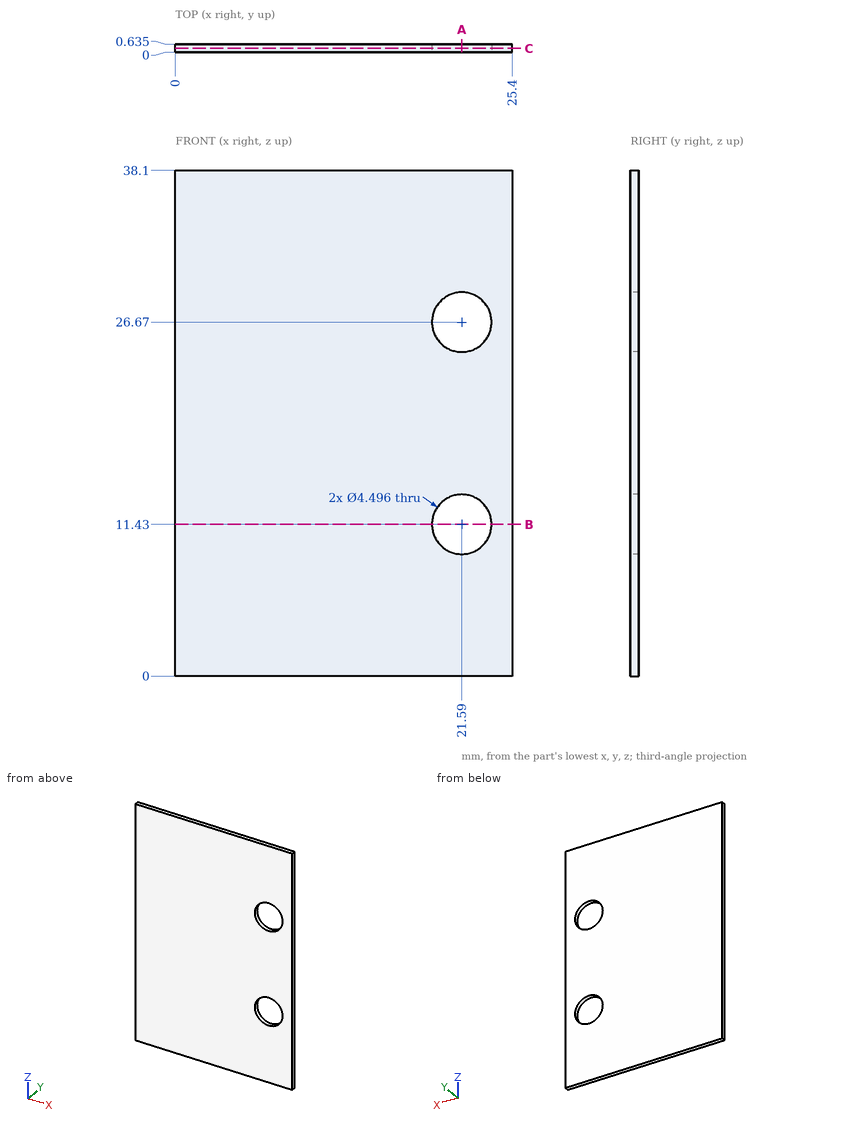
Check sheet for the drawn part. Datum: minimum x, y, z corner. Units: mm. Coordinates: 2 decimals unless noted, no trailing zeros. Order: outer loops, then holes, each group sorted by start corner. A loop starts at its lowest first (then second) coordinate and runs counter-clockwise, first axis right, second up. Notation, with made-up numbers: M 58.5,4 L 100.5,4 A5 ccw 100.5,10 Z; hole C 74.5,15 d9. An arc over 180 degrees is marked long. One line per question, with ' | ' between items. Start each with the question number.
Item 1: Cross-section at B-B on z = 11.43. Enter the section's corners in (x, y) (1 decimal).
Item 2: Cross-section at C-C on y = 0.3. Enter the section's corners in (x, z), then the cut area to 3 significant figures.
Item 3: Material ranges on L1, parallel to Z at x = 21.59, y = 0.55; L2, parallel to X at y = 0.3, z = 11.43; L3, parallel to Z at x = 22, y = 0.3, recorded low to high. Write a range as [from, to].
Item 4: Gauge pin test, flat end, axial feed: pin 1 (4 mm diameter, centred on x = 21.59, z = 11.43, fed in from -Y). Record the tip position at first contact, or that the pin passes through.
Item 5: Cross-section at A-A on x = 21.59. Enter the section's corners in (y, z) (1 decimal).
Findings:
1) outline: M 0,0 L 19.3,0 L 19.3,0.6 L 0,0.6 Z; M 23.8,0 L 25.4,0 L 25.4,0.6 L 23.8,0.6 Z
2) outline: M 0,0 L 25.4,0 L 25.4,38.1 L 0,38.1 Z; hole C 21.59,11.43 d4.5; hole C 21.59,26.67 d4.5 | area: 936 mm²
3) L1: z = [0, 9.18], [13.68, 24.42], [28.92, 38.1] | L2: x = [0, 19.34], [23.84, 25.4] | L3: z = [0, 9.22], [13.64, 24.46], [28.88, 38.1]
4) pin 1: passes through
5) outline: M 0,0 L 0.6,0 L 0.6,9.2 L 0,9.2 Z; M 0,13.7 L 0.6,13.7 L 0.6,24.4 L 0,24.4 Z; M 0,28.9 L 0.6,28.9 L 0.6,38.1 L 0,38.1 Z
